Input: dimensioned drawing with shaded views. Units: mm. Origin: part minimum x, y, z. Give positions to 0.01 mm unless a question says otherwise; leave off trailing zeros. Write each loop counter-clockwise with the first axis right and the second up, starting at its lowest first coordinate (ties: lowest second). Pieces come first, ordered by that corner, then holes. Notation, with made-up numbers: M 77.25,79.25 L 117.25,79.25 A29 cw 117.25,109.25 Z; hole C 56,41 d9. An arc over 180 degrees is marked long. Answer as a JSON object with one key per item and string values.
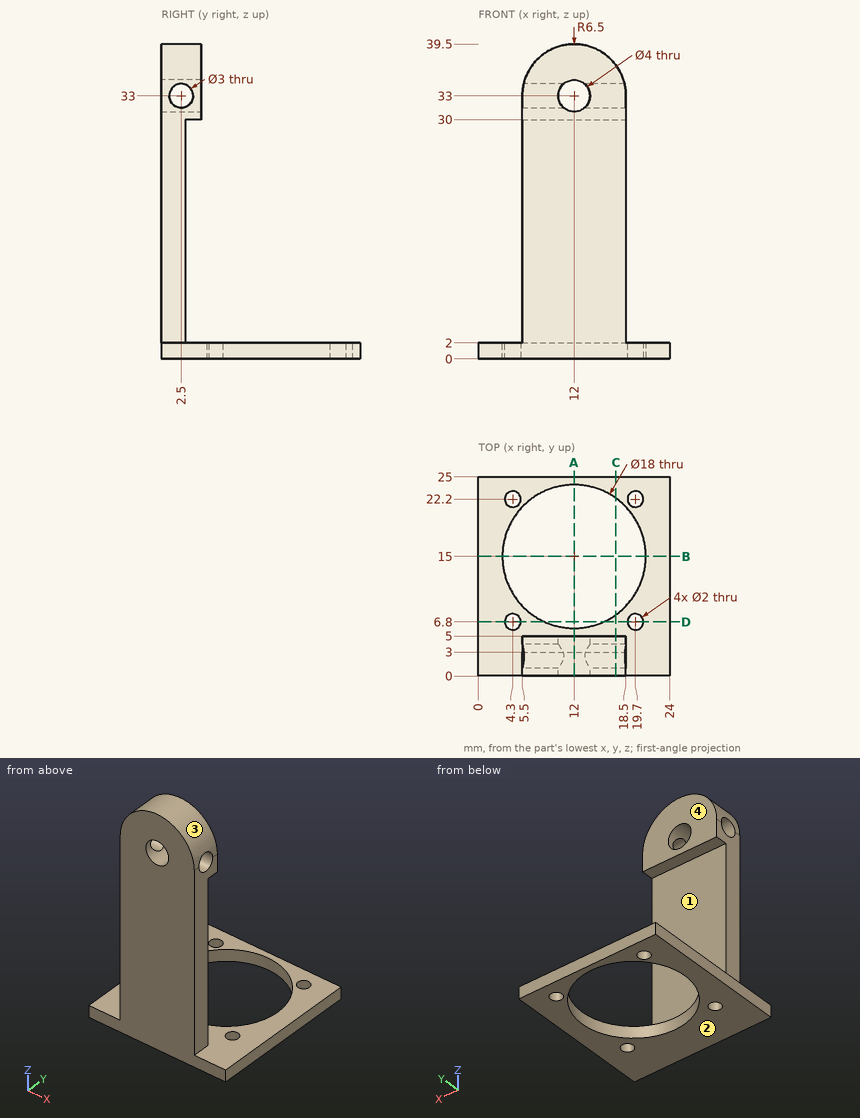
1) Cut plane B-B on y = 15. Return loops of the section in (x, z), and give its area (3 significant figures).
Geometry check:
{"outline": "M 0,0 L 3,0 L 3,2 L 0,2 Z; M 21,0 L 24,0 L 24,2 L 21,2 Z", "area": "12.0 mm2"}
2) Contact query for flat-ended pins moving along their axis: P1, Ø3, axis at x = 12, z = 33, coming from the +Y side; P2, Ø4, axis at x = 13.5, y = 7.5, coming from the +Z side; P3, Ø10.5, axis at x = 14.5, z = 22, coming from the +Y side; P4, Ø5, axis at y = 2.5, z = 33, coming from the -X side. Output: stop coordinate, or through.
Geometry check:
{"P1": "passes through", "P2": "stops at z = 2", "P3": "stops at y = 3", "P4": "stops at x = 5.5"}
3) Cut plane D-D on y = 6.8. Return loops of the section in (x, z).
Geometry check:
{"outline": "M 0,0 L 3.3,0 L 3.3,2 L 0,2 Z; M 5.3,0 L 8.29,0 L 8.29,2 L 5.3,2 Z; M 15.71,0 L 18.7,0 L 18.7,2 L 15.71,2 Z; M 20.7,0 L 24,0 L 24,2 L 20.7,2 Z"}
4) Pull-direction query (Z, two-part tool) for the marked faces 1, 2, 3 and 4; classes: pulls with the +Z half, pulls with the -Z half, needs draft (parallel to the pull), parting line crosses it, or undercut.
Geometry check:
{"face 1": "undercut", "face 2": "pulls with the -Z half", "face 3": "pulls with the +Z half", "face 4": "needs draft"}
5) Line query: line 1 (Y direction, x = 19.7, z = 0.75); line 2 (Z direction, x = 22.25, y = 19.5); line 3 (Y direction, x = 9.25, z = 33). Output: solid intervals per line, ascending. Write a range as from..to.
Geometry check:
{"line 1": "y = 0..5.8, 7.8..10.34, 19.66..21.2, 23.2..25", "line 2": "z = 0..2", "line 3": "y = 0..1, 4..5"}
6) Cut plane C-C on x = 17.25. Return loops of the section in (y, z).
Geometry check:
{"outline": "M 0,0 L 7.69,0 L 7.69,2 L 3,2 L 3,30 L 5,30 L 5,36.83 L 0,36.83 Z; M 22.31,0 L 25,0 L 25,2 L 22.31,2 Z; hole C 2.5,33 d3"}
7) Cut plane A-A on x = 12. Return loops of the section in (y, z), and give its area (4 significant figures).
Geometry check:
{"outline": "M 0,0 L 6,0 L 6,2 L 3,2 L 3,30 L 5,30 L 5,31 L 0,31 Z; M 0,35 L 5,35 L 5,39.5 L 0,39.5 Z; M 24,0 L 25,0 L 25,2 L 24,2 Z", "area": "125.5 mm2"}
